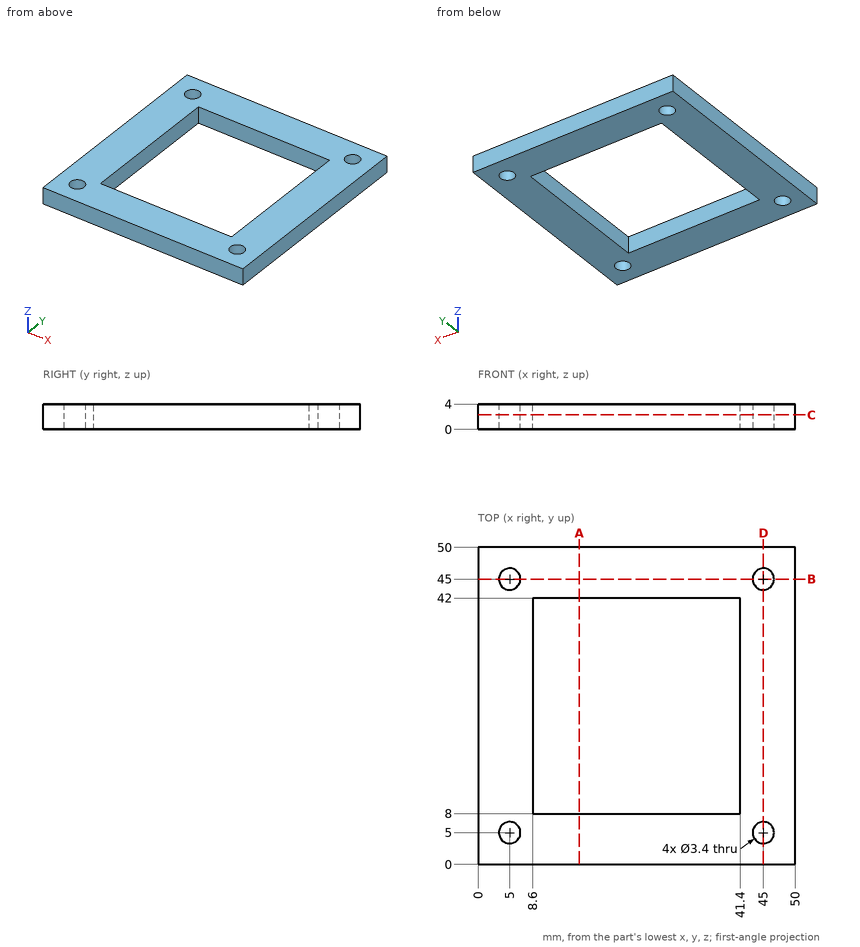
Design review of the part shown in the three views and the two pictorial views. Dimensions are in mm from the part's minimum x, y and z. Coordinates: 2 decimals unless noted, no trailing zeros. Write each loop counter-clockwise with the first axis right and the second up, starting at its lowest first coordinate (ties: lowest second). Pieces come first, ordered by that corner, then holes.
1) Clearance check with flat-ended pins moving along their axes: pin 1 Ø1.2 at (x, z) = (22.5, 1) entering from -Y; pin 2 Ø3 at (x, y) = (5, 45) entering from +Z. State where each tip first meets the part, or that it passes through.
2) We need section A-A on x = 16. State the section outline as (y, z) points.
3) We need section B-B on y = 45. State the section outline as (x, z) points.
4) We need section C-C on z = 2.3. State the section outline as (x, y) points.
5) To check wall thickness, follow probe 1 along Y at (x, z) = (45, 1.6); probe 2 along X at (y, z) = (30, 1.95); probe 3 along Y at (x, z) = (23.5, 0.35). State the ranges of each line that lie inside material, in increasing order.
Answer list:
1. pin 1: stops at y = 0
1. pin 2: passes through
2. outline: (0, 0) - (8, 0) - (8, 4) - (0, 4) - close; (42, 0) - (50, 0) - (50, 4) - (42, 4) - close
3. outline: (0, 0) - (3.3, 0) - (3.3, 4) - (0, 4) - close; (6.7, 0) - (43.3, 0) - (43.3, 4) - (6.7, 4) - close; (46.7, 0) - (50, 0) - (50, 4) - (46.7, 4) - close
4. outline: (0, 0) - (50, 0) - (50, 50) - (0, 50) - close; hole circle Ø3.4 at (5, 5); hole circle Ø3.4 at (5, 45); hole (8.6, 8) - (41.4, 8) - (41.4, 42) - (8.6, 42) - close; hole circle Ø3.4 at (45, 5); hole circle Ø3.4 at (45, 45)
5. probe 1: y = 0 to 3.3, 6.7 to 43.3, 46.7 to 50
5. probe 2: x = 0 to 8.6, 41.4 to 50
5. probe 3: y = 0 to 8, 42 to 50
